Read the model definition and answer for the solid it produces. Units are mm, in the model's axes. A direction names the side the tool comes from. Coordinates: 2 decimals unless noted, no trailing zeros. Write each loop counter-clockwise with the first axis right and the second up, starting at its lowest first coordinate (ties: lowest second). Pieces come first, ordered by that corner, then holes. Notation, with made-up numbers: (89, 64.25) - (120, 64.25) arc R25 ccw to (120, 89.25) - close; hole circle Ø4 at (-2, 32). An arc over 180 degrees is marked (long way). Use a Markdown table: item, result.
from build123d import *

# Parameters (mm, degrees)
CHAMFER1_SIZE = 0.4
SKETCH2_W     = 1.1
SKETCH2_H     = 0.2


with BuildPart() as part:
    # Sketch1 → Revolve1 (revolve)
    with BuildSketch(Plane(origin=(0, 0, 0), x_dir=(1, 0, 0), z_dir=(0, 1, 0)), mode=Mode.PRIVATE) as revolve1_sk:
        Polygon((0, 0), (0, 10), (10.5, 10), (10.5, 7), (11.5, 7), (11.5, 5), (19.5, 5), (19.5, 0), align=None)
    revolve(revolve1_sk.sketch.rotate(Axis((0, 0, 0), (1, 0, 0)), 180), axis=Axis((0, 0, 0), (1, 0, 0)))

    # Chamfer1
    chamfer1_edges = [part.edges().sort_by_distance(p)[0] for p in [
        (19.5, 0, -5),
        (10.5, 0, -10),
        (0, 0, -10),
    ]]
    chamfer(chamfer1_edges, length=CHAMFER1_SIZE)

    # Sketch2 → Cut-Revolve1 (revolve, cut)
    with BuildSketch(Plane(origin=(0, 0, 0), x_dir=(1, 0, 0), z_dir=(0, 1, 0)), mode=Mode.PRIVATE) as cut_revolve1_sk:
        with Locations((17.25, 4.9)):
            Rectangle(SKETCH2_W, SKETCH2_H)
    revolve(cut_revolve1_sk.sketch.rotate(Axis((11.5, 0, 0), (1, 0, 0)), 180), axis=Axis((11.5, 0, 0), (1, 0, 0)), mode=Mode.SUBTRACT)


solid = part.part
(1) Each of these flat-tipped pins is pushed along its axis until it touches: P1, Ø1, axis at y = -3, z = 8, coming from the +X side; P2, Ø1, axis at x = 11.5, y = -3, coming from the -Z side; P3, Ø5, axis at x = 2.5, z = 4.5, coming from the -Y side; P4, Ø1, axis at x = 14.5, z = 6, coming from the -Y side (3 decimals). Where does it stop, or does it pass through?
Report:
| item | result |
|---|---|
| P1 | stops at x = 10.5 |
| P2 | stops at z = -6.54 |
| P3 | stops at y = -9.8 |
| P4 | passes through |
(2) A cutting plane is placed at A-A, the plane y = 0. Write down the section's boundary in (x, z).
Report:
| item | result |
|---|---|
| outline | (0, -9.6) - (0.4, -10) - (10.1, -10) - (10.5, -9.6) - (10.5, -7) - (11.5, -7) - (11.5, -5) - (16.7, -5) - (16.7, -4.8) - (17.8, -4.8) - (17.8, -5) - (19.1, -5) - (19.5, -4.6) - (19.5, 4.6) - (19.1, 5) - (17.8, 5) - (17.8, 4.8) - (16.7, 4.8) - (16.7, 5) - (11.5, 5) - (11.5, 7) - (10.5, 7) - (10.5, 9.6) - (10.1, 10) - (0.4, 10) - (0, 9.6) - close |
(3) A cutting plane is placed at D-D, the plane x = 14. Write down the section's boundary in (y, z).
Report:
| item | result |
|---|---|
| outline | circle Ø10 at (0, 0) |
(4) Straight lines are drawn through the part: L1, parallel to X at y = 5.25, z = 5.75; L2, parallel to X at y = 1.75, z = -5.5; L3, parallel to Z at x = 13.75, y = 1.5. For each, find the intervals that lie inside material, in ascending order.
Report:
| item | result |
|---|---|
| L1 | x = 0 to 10.5 |
| L2 | x = 0 to 11.5 |
| L3 | z = -4.77 to 4.77 |
(5) The mould has two halves that part along X. Classify faces 1 (the cylindrical face through (18, 0, -5)), 2 (the flat face through (11.5, -5, -2)), 3 (the cylindrical face through (17.26, -4.05, 2.58)): pulls with the +X half, pulls with the -X half, needs draft (parallel to the pull), parting line crosses it, or undercut.
Report:
| item | result |
|---|---|
| face 1 | needs draft |
| face 2 | pulls with the +X half |
| face 3 | undercut |
(6) A cutting plane is placed at C-C, the plane x = 6.75. Write down the section's boundary in (y, z), and give its area (3 significant figures).
Report:
| item | result |
|---|---|
| outline | circle Ø20 at (0, 0) |
| area | 314 mm² |
(7) For faces 4 (the flat face through (19.5, 0, 0)), 5 (the flat face through (10.5, 6, 4)), determine the directions among +Z, -Z, +X, -X, +Y, -Y from which every point of the face is accessible in a straight line to the end or side of a thin tool.
Report:
| item | result |
|---|---|
| face 4 | +Z, -Z, +X, +Y, -Y |
| face 5 | +X |
